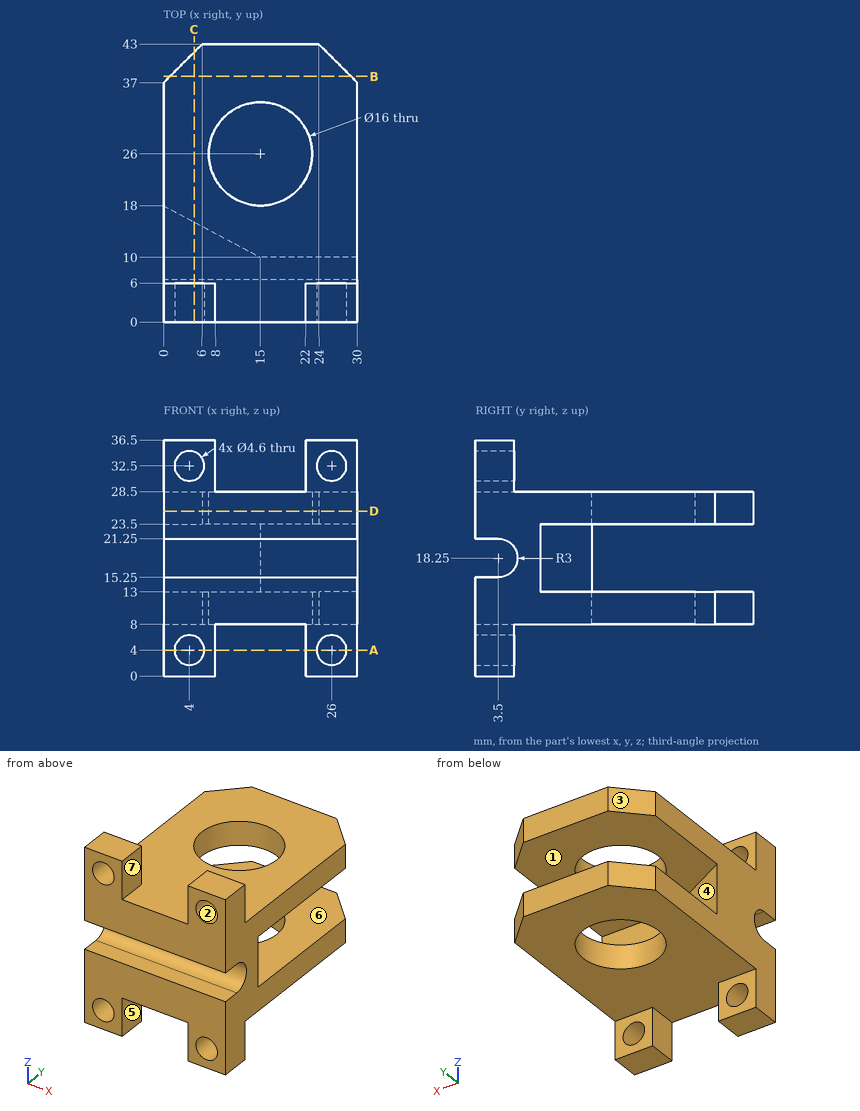
Job drawing, mm, ordinate dimensions from the low corner. One solid piece. A direction names the side the tool comes from. Give positions to 0.01 mm unless a question says otherwise; leave off trailing zeros. Order: outer loops, then holes, each group sorted by start corner. A loop starts at its lowest first (then second) coordinate and runs counter-clockwise, first axis right, second up. Notation, with made-up numbers: M -28.5,14 L 14.5,14 A10 ccw 14.5,23 Z; hole C 72.25,39.25 d9. An arc over 180 degrees is marked long. Return JSON: item names as keys, results as strings.
Q1. Band-saw the part on D-D (z = 25.5). Give the cut face in (x, y), then the cut area to 3 significant figures.
Answer list:
{"outline": "M 0,0 L 30,0 L 30,37 L 24,43 L 6,43 L 0,37 Z; hole C 15,26 d16", "area": "1,050 mm^2"}
Q2. Wall check: probe 1 along Z at (x, y) = (1.5, 28); probe 2 along X at (y, z) = (26, 11.9); probe 3 along X at (y, z) = (1.5, 4). Give the ranges that are in metal, low to high. Write a range as from..to.
Answer list:
{"probe 1": "z = 8..13, 23.5..28.5", "probe 2": "x = 0..7, 23..30", "probe 3": "x = 0..1.7, 6.3..8, 22..23.7, 28.3..30"}
Q3. Two-plate mould, pull along X, no slides. Class the marked faces 1, 2, 3 and 4: pulls with the +X half, pulls with the -X half, needs draft (parallel to the pull), parting line crosses it, or undercut.
Answer list:
{"face 1": "needs draft", "face 2": "undercut", "face 3": "pulls with the -X half", "face 4": "pulls with the +X half"}
Q4. Band-saw the part on B-B (y = 38). Give the cut face in (x, z), then the cut area to 3 significant figures.
Answer list:
{"outline": "M 1,8 L 29,8 L 29,13 L 1,13 Z; M 1,23.5 L 29,23.5 L 29,28.5 L 1,28.5 Z", "area": "280 mm^2"}
Q5. Band-saw the part on C-C (x = 4.75). Give the cut face in (y, z).
Answer list:
{"outline": "M 0,0 L 6,0 L 6,1.83 L 0,1.83 Z; M 0,6.17 L 6,6.17 L 6,8 L 41.75,8 L 41.75,13 L 15.47,13 L 15.47,23.5 L 41.75,23.5 L 41.75,28.5 L 6,28.5 L 6,30.33 L 0,30.33 L 0,21.25 L 3.5,21.25 A3 cw 3.5,15.25 L 0,15.25 Z; M 0,34.67 L 6,34.67 L 6,36.5 L 0,36.5 Z"}
Q6. 3-axis set-ups, long thin cutter, end or side, ignore diameter. For the marked faces 5, 6 and 7: which of +Z, -Z, +X, -X, +Y, -Y reach the whole face in a straight line?
Answer list:
{"face 5": "-Z, +Y, -Y", "face 6": "+X, +Y", "face 7": "+Z, +Y, -Y"}
Q7. Band-saw the part on A-A (z = 4). Give the cut face in (x, y), then the cut area to 3 significant figures.
Answer list:
{"outline": "M 0,0 L 1.7,0 L 1.7,6 L 0,6 Z; M 6.3,0 L 8,0 L 8,6 L 6.3,6 Z; M 22,0 L 23.7,0 L 23.7,6 L 22,6 Z; M 28.3,0 L 30,0 L 30,6 L 28.3,6 Z", "area": "40.8 mm^2"}
Q8. Flat gauge pins, fed straight in: pin 1 (3 mm diameter, centred on x = 26, z = 32.5, fed in from -Y); pin 2 (1 mm diameter, centred on x = 8, y = 13, fed in from -Z); pin 3 (4 mm diameter, centred on x = 25.5, z = 32, fed in from +Y); pin 4 (5 mm diameter, centred on x = 25.5, y = 38, fed in from +Z). Where does each tip first touch, or does it go through?
Answer list:
{"pin 1": "passes through", "pin 2": "stops at z = 8", "pin 3": "stops at y = 6", "pin 4": "stops at z = 28.5"}
